```python
from build123d import *

# Parameters (mm, degrees)
SKETCH1_R           = 2.5
SKETCH1_R_2         = 11
BOSS_EXTRUDE1_DEPTH = 6.35
FILLET1_R           = 5
FILLET2_R           = 3


with BuildPart() as part:
    # Sketch1 → Boss-Extrude1 (new body)
    with BuildSketch(Plane.XY):
        Polygon((20, 61.824817518), (-60, 61.824817518), (-140, -58.175182482), (-140, -78.175182482), (20, -78.175182482), align=None)
        with Locations((-50, -48.175182482)):
            Circle(SKETCH1_R, mode=Mode.SUBTRACT)
        with Locations((-50, -28.175182482)):
            Circle(SKETCH1_R, mode=Mode.SUBTRACT)
        with Locations((-50, -8.175182482)):
            Circle(SKETCH1_R, mode=Mode.SUBTRACT)
        with Locations((-50, 11.824817518)):
            Circle(SKETCH1_R, mode=Mode.SUBTRACT)
        with Locations((-50, 31.824817518)):
            Circle(SKETCH1_R, mode=Mode.SUBTRACT)
        with Locations((-50, 51.824817518)):
            Circle(SKETCH1_R, mode=Mode.SUBTRACT)
        with Locations((-30, -48.175182482)):
            Circle(SKETCH1_R, mode=Mode.SUBTRACT)
        with Locations((-30, 51.824817518)):
            Circle(SKETCH1_R, mode=Mode.SUBTRACT)
        with Locations((-10, 1.824817518)):
            Circle(SKETCH1_R_2, mode=Mode.SUBTRACT)
        with Locations((-30, -68.175182482)):
            Circle(SKETCH1_R, mode=Mode.SUBTRACT)
        with Locations((-50, -68.175182482)):
            Circle(SKETCH1_R, mode=Mode.SUBTRACT)
        with Locations((-70, -68.175182482)):
            Circle(SKETCH1_R, mode=Mode.SUBTRACT)
        with Locations((-90, -68.175182482)):
            Circle(SKETCH1_R, mode=Mode.SUBTRACT)
        with Locations((-110, -68.175182482)):
            Circle(SKETCH1_R, mode=Mode.SUBTRACT)
        with Locations((-130, -68.175182482)):
            Circle(SKETCH1_R, mode=Mode.SUBTRACT)
    extrude(amount=BOSS_EXTRUDE1_DEPTH)

    # Fillet1
    fillet1_edges = [part.edges().sort_by_distance(p)[0] for p in [
        (-140, -58.175182482, 3.175),
        (-60, 61.824817518, 3.175),
    ]]
    fillet(fillet1_edges, radius=FILLET1_R)

    # Fillet2
    fillet2_edges = [part.edges().sort_by_distance(p)[0] for p in [
        (20, -78.175182482, 3.175),
        (-140, -78.175182482, 3.175),
        (20, 61.824817518, 3.175),
    ]]
    fillet(fillet2_edges, radius=FILLET2_R)


solid = part.part
```
Read the model definition and answer for the solid it produces. Units are mm, in the model's axes. Coordinates: 2 decimals unless noted, no trailing zeros. Write each loop counter-clockwise with the first axis right and the second up, starting at its lowest first coordinate (ties: lowest second). Pieces come first, ordered by that corner, then holes. Notation, with made-up numbers: (51.25, 0) -> (64.25, 0) arc R28 ccw to (64.25, 28) -> close; hole circle Ø2 at (68.25, 38.25). An arc over 180 degrees is marked (long way). Answer as a JSON object with one key per item and string values.
Q1. The part is cut by section A-A on x = -50. Give the number of separate pieces and of enclosed holes in the cut face, then the cut area to 3 significant figures.
The answers:
{"separate pieces": "8", "enclosed holes": "0", "area": "667 mm2"}
Q2. The part is cut by section C-C on y = 7. Give the vertices of the cut face in (x, z).
The answers:
{"outline": "(-96.55, 0) -> (-19.71, 0) -> (-19.71, 6.35) -> (-96.55, 6.35) -> close; (-0.29, 0) -> (20, 0) -> (20, 6.35) -> (-0.29, 6.35) -> close"}
Q3. Determine the mould class of faces 1 (the cylindrical face through (-59.65, 61.25, 3.22)), 2 (the cylindrical face through (-90.542, -70.616, 3.131)), 3 (the flat face through (20, -9, 3)) for opening direction X: pulls with the +X half, pulls with the -X half, needs draft (parallel to the pull), parting line crosses it, or undercut.
The answers:
{"face 1": "pulls with the -X half", "face 2": "undercut", "face 3": "pulls with the +X half"}
Q4. The part is cut by section B-B on x = -30. Give the vertices of the cut face in (y, z).
The answers:
{"outline": "(-78.18, 0) -> (-70.68, 0) -> (-70.68, 6.35) -> (-78.18, 6.35) -> close; (-65.68, 0) -> (-50.68, 0) -> (-50.68, 6.35) -> (-65.68, 6.35) -> close; (-45.68, 0) -> (49.32, 0) -> (49.32, 6.35) -> (-45.68, 6.35) -> close; (54.32, 0) -> (61.82, 0) -> (61.82, 6.35) -> (54.32, 6.35) -> close"}
Q5. Flat-ended cylindrical pins translate along their axes: pin 1 Ø1 at (x, z) = (-80, 3.5) entering from +Y; pin 2 Ø1.5 at (y, z) = (-52, 4.5) entering from -X. Find the tip coordinate at first contact, or state that the pin passes through.
The answers:
{"pin 1": "stops at y = 32.57", "pin 2": "stops at x = -136.38"}
Q6. Consider line 1 (Y direction, x = -30, z = 1.5); line 2 (X direction, y = -49, z = 3); line 3 (X direction, y = 53, z = 2). Determine where each line is inside the solid, lowest interval first. Write a range as [from, to].
The answers:
{"line 1": "y = [-78.18, -70.68], [-65.68, -50.68], [-45.68, 49.32], [54.32, 61.82]", "line 2": "x = [-133.88, -52.36], [-47.64, -32.36], [-27.64, 20]", "line 3": "x = [-65.88, -52.21], [-47.79, -32.21], [-27.79, 20]"}
